Part model, mm, in its own coordinate system. Give positions to 0.01 mm unless a question says otherwise; leave off trailing zeros. Loops run counter-clockwise (first coordinate to the right, second up) from the corner with the lowest first, then second, coordinate; pieces in that order, holes last. Notation, with made-up numbers: M -4.5,-31 L 12.5,-31 A21 ccw 12.5,-6 Z; hole C -6.75,-23.5 d5. An arc over 180 degrees is marked long. Put each result on its own line as item: value. Start each with the question number.
```python
from build123d import *

# Parameters (mm, degrees)
F0_R     = 31
F1_DEPTH = 45
F2_R     = 6.25
F3_DEPTH = 51
F4_R     = 5.5
F5_DEPTH = 45
F6_R     = 5.5
F7_DEPTH = 45
F8_R     = 2
F9_DEPTH = 45


with BuildPart() as f1:
    # F0 (on Top) → F1 (new body)
    with BuildSketch(Plane.XY):
        Circle(F0_R)
    extrude(amount=F1_DEPTH)

    # F2 (on face) → F3 (cut)
    with BuildSketch(Plane(origin=(0, 0, 0), x_dir=(1, 0, 0), z_dir=(0, 0, -1))):
        Circle(F2_R)
    extrude(amount=-F3_DEPTH, mode=Mode.SUBTRACT)

    # F4 (on face) → F5 (cut)
    with BuildSketch(Plane(origin=(0, 0, 0), x_dir=(1, 0, 0), z_dir=(0, 0, -1))):
        with Locations((0, 24)):
            Circle(F4_R)
        with Locations((-12, 20.78461)):
            Circle(F4_R)
        with Locations((-20.78461, 12)):
            Circle(F4_R)
        with Locations((-24, 0)):
            Circle(F4_R)
        with Locations((-20.78461, -12)):
            Circle(F4_R)
        with Locations((-12, -20.78461)):
            Circle(F4_R)
        with Locations((0, -24)):
            Circle(F4_R)
        with Locations((12, -20.78461)):
            Circle(F4_R)
        with Locations((20.78461, -12)):
            Circle(F4_R)
        with Locations((24, 0)):
            Circle(F4_R)
        with Locations((20.78461, 12)):
            Circle(F4_R)
        with Locations((12, 20.78461)):
            Circle(F4_R)
    extrude(amount=-F5_DEPTH, mode=Mode.SUBTRACT)

    # F2 (on face) + F6 (on face) → F7 (cut)
    with BuildSketch(Plane(origin=(0, 0, 0), x_dir=(1, 0, 0), z_dir=(0, 0, -1))):
        Circle(F2_R)
    with BuildSketch(Plane(origin=(0, 0, 0), x_dir=(1, 0, 0), z_dir=(0, 0, -1))):
        with Locations((-12.557036, 3.364648)):
            Circle(F6_R)
        with Locations((-9.192388, -9.192388)):
            Circle(F6_R)
        with Locations((3.364648, -12.557036)):
            Circle(F6_R)
        with Locations((12.557036, -3.364648)):
            Circle(F6_R)
        with Locations((9.192388, 9.192388)):
            Circle(F6_R)
        with Locations((-3.364648, 12.557036)):
            Circle(F6_R)
    extrude(amount=-F7_DEPTH, mode=Mode.SUBTRACT)

    # F8 (on face) → F9 (cut)
    with BuildSketch(Plane(origin=(0, 0, 0), x_dir=(1, 0, 0), z_dir=(0, 0, -1))):
        with Locations((4.399924, 16.420739)):
            Circle(F8_R)
        with Locations((-12.020815, 12.020815)):
            Circle(F8_R)
        with Locations((-16.420739, -4.399924)):
            Circle(F8_R)
        with Locations((-4.399924, -16.420739)):
            Circle(F8_R)
        with Locations((12.020815, -12.020815)):
            Circle(F8_R)
        with Locations((16.420739, 4.399924)):
            Circle(F8_R)
    extrude(amount=-F9_DEPTH, mode=Mode.SUBTRACT)


solid = f1.part
```
1) Pin check, flat tips, straight feed: pin 1 Ø1.5 at (x, z) = (-6.5, 16) entering from -Y; pin 2 Ø8 at (x, z) = (3.5, 31) entering from -Y; pin 3 Ø8 at (x, z) = (23, 9.5) entering from -Y; pin 4 Ø6.5 at (x, y) = (3.36, 12.56) entering from -Z. Stop position of each tip, or through.
2) Mould opens along Y. For faces 1 (the cylindrical face through (-9.462, -15.905, 22.185)), 2 (the flat face through (6.5, 0.4, 45)) say: +Y half, -Y half, draft (parallel to the pull), parting line (faces both ways), or undercut.
3) Band-saw the part on A-A on x = 12. Give the cut face in (y, z), then the cut area to 3 significant figures.
4) Band-saw the part on B-B on y = -24. Give the cut face in (x, z).
5) Band-saw the part on C-C on x = 20. Give the cut face in (y, z).
6) Band-saw the part on D-D on z = 12. State how many separate pieces and enclosed holes the cut face has, then the cut area to 3 significant figures.
7) Wall check: L1, parallel to Y at x = 19.5, z = 32; L2, parallel to Y at x = -13, z = 5; L3, parallel to X at y = 12, z = 14.5. Give the ranges that are in metal, low to high.
Evaluation:
1. pin 1: y = -30.46
1. pin 2: y = -31
1. pin 3: y = -24.49
1. pin 4: through
2. face 1: undercut
2. face 2: draft
3. outline: M -28.58,0 L -26.28,0 L -26.28,45 L -28.58,45 Z; M -15.28,0 L -13.92,0 L -13.92,45 L -15.28,45 Z; M -4.46,0 L -2.11,0 L -2.11,45 L -4.46,45 Z; M 8.84,0 L 10.02,0 L 10.02,45 L 8.84,45 Z; M 14.02,0 L 15.28,0 L 15.28,45 L 14.02,45 Z; M 26.28,0 L 28.58,0 L 28.58,45 L 26.28,45 Z
3. area: 484 mm2
4. outline: M -19.62,0 L -16.46,0 L -16.46,45 L -19.62,45 Z; M -7.54,0 L -5.5,0 L -5.5,45 L -7.54,45 Z; M 5.5,0 L 7.54,0 L 7.54,45 L 5.5,45 Z; M 16.46,0 L 19.62,0 L 19.62,45 L 16.46,45 Z
5. outline: M -23.69,0 L -17.44,0 L -17.44,45 L -23.69,45 Z; M -6.56,0 L -3.77,0 L -3.77,45 L -6.56,45 Z; M 3.77,0 L 6.56,0 L 6.56,45 L 3.77,45 Z; M 17.44,0 L 23.69,0 L 23.69,45 L 17.44,45 Z
6. separate pieces: 1
6. enclosed holes: 25
6. area: 1,110 mm2
7. L1: -24.1 to -17.35, -6.65 to -3.16, 3.16 to 6.65, 17.35 to 24.1
7. L2: -28.14 to -26.19, -15.38 to -13.76, -10.28 to -8.85, 2.12 to 5.22, 13.16 to 15.38, 26.19 to 28.14
7. L3: -28.58 to -26.28, -15.28 to -13.92, -4.46 to -2.11, 8.84 to 10.02, 14.02 to 15.28, 26.28 to 28.58
